```python
from build123d import *

# Parameters (mm, degrees)
CHAMFER1_SIZE      = 0.5
SKETCH2_R          = 6
CUT_EXTRUDE1_DEPTH = 0.5


with BuildPart() as part:
    # Sketch1 → Revolve1 (revolve)
    with BuildSketch(Plane.XY):
        Polygon((2.5, 0), (2.5, 16), (8, 16), (8, 14.5), (6.12, 14.5), (6.12, 7.4), (8, 7.4), (8, 0), align=None)
    revolve(axis=Axis((0, 0, 0), (0, 1, 0)))

    # Chamfer1
    chamfer1_edges = [part.edges().sort_by_distance(p)[0] for p in [
        (-8, 7.4, 0),
        (-8, 14.5, 0),
    ]]
    chamfer(chamfer1_edges, length=CHAMFER1_SIZE)

    # Sketch2 → Cut-Extrude1 (cut)
    with BuildSketch(Plane(origin=(0, 16, 0), x_dir=(1, 0, 0), z_dir=(0, 1, 0))):
        Circle(SKETCH2_R)
    extrude(amount=-CUT_EXTRUDE1_DEPTH, mode=Mode.SUBTRACT)


solid = part.part
```
Model file for the job. Use its own axes, mm. A direction names the side the tool comes from. Round coordinates to 2 decimals unless told otherwise and drop trailing zeros. Write each loop counter-clockwise with the first axis right and the second up, starting at its lowest first coordinate (ties: lowest second). Pieces come first, ordered by that corner, then holes. Notation, with made-up numbers: M 5,-30 L 27,-30 A9 cw 27,-21 Z; hole C 9,-20 d7. An arc over 180 degrees is marked long. Put each result on its own line as item: value.
Item 1: Cut at C-C (y = 12.5). List the corners of the cut face in (x, z).
Responses:
outline: C 0,0 d12.24; hole C 0,0 d5
Item 2: Tool access for faces 1 (the flat face through (3, 15.5, 0)), 2 (the flat face through (3, 7.4, 6)), 3 (the cylindrical face through (-1.73, 15.49, 7.81)): list every direction of +Z, -Z, +X, -X, +Y, -Y with a clear straight run to the whole face (end or side of a thin tool).
Responses:
face 1: +Y
face 2: none
face 3: +Y, -Y
Item 3: Mould opens along Z. For faces 4 (the cylindrical face through (-1.73, 3.4, 7.81)), 5 (the cylindrical face through (-0.54, 7.86, 2.44)), 6 (the flat face through (-2, 0, 2)) say: +Z half, -Z half, draft (parallel to the pull), parting line (faces both ways), or undercut.
Responses:
face 4: parting line
face 5: undercut
face 6: draft
Item 4: Cut at A-A (z = 0). List the corners of the cut face in (x, y).
Responses:
outline: M -8,0 L -2.5,0 L -2.5,15.5 L -6,15.5 L -6,16 L -8,16 L -8,15 L -7.5,14.5 L -6.12,14.5 L -6.12,7.4 L -7.5,7.4 L -8,6.9 Z; M 2.5,0 L 8,0 L 8,6.9 L 7.5,7.4 L 6.12,7.4 L 6.12,14.5 L 7.5,14.5 L 8,15 L 8,16 L 6,16 L 6,15.5 L 2.5,15.5 Z
Item 5: Cut at D-D (y = 1.5). List the corners of the cut face in (x, z).
Responses:
outline: C 0,0 d16; hole C 0,0 d5
Item 6: Probe L1, parallel to X at y = 4.75, z = 0; L2, parallel to X at y = 15.6, z = 0. List the from-to ranges inside material, lowest first. Write a range as from..to.
Responses:
L1: -8..-2.5, 2.5..8
L2: -8..-6, 6..8
Item 7: Cut at B-B (x = 0). List the corners of the cut face in (y, z), and give its area (3 significant figures).
Responses:
outline: M 0,-8 L 6.9,-8 L 7.4,-7.5 L 7.4,-6.12 L 14.5,-6.12 L 14.5,-7.5 L 15,-8 L 16,-8 L 16,-6 L 15.5,-6 L 15.5,-2.5 L 0,-2.5 Z; M 0,2.5 L 15.5,2.5 L 15.5,6 L 16,6 L 16,8 L 15,8 L 14.5,7.5 L 14.5,6.12 L 7.4,6.12 L 7.4,7.5 L 6.9,8 L 0,8 Z
area: 145 mm²
Item 8: Flat gauge pins, fed straight in: P1, Ø3, axis at y = 9.5, z = -4.5, coming from the -X side; P2, Ø1.5, axis at x = 4, y = 13, coming from the -Z side; P3, Ø4.5, axis at x = -1.5, z = -1, coming from the -Y side; P4, Ø6, axis at x = -1.5, z = 2.5, coming from the +Y side. Where does each tip first touch, or does it go through?
Responses:
P1: x = -5.33
P2: z = -5.19
P3: y = 0
P4: y = 15.5
